Model file for the job. Use its own axes, mm. A direction names the side the tool comes from. Coordinates: 2 decimals unless noted, no trailing zeros. Loops run counter-clockwise (first coordinate to the right, second up) from the corner with the lowest first, then second, coordinate; pieces in that order, holes last. Notation, with made-up numbers: (2, 4.5) -> (6, 4.5) arc R33 ccw to (6, 42.5) -> close; hole circle Ø6 at (64.5, -21). An arc over 180 degrees is marked (long way). Use one line per item in the form item = value.
```python
from build123d import *

# Parameters (mm, degrees)
SKETCH1_W           = 100
SKETCH1_H           = 20
BOSS_EXTRUDE1_DEPTH = 3
SKETCH2_W           = 4.785100676
SKETCH2_H           = 2.523053084
CUT_EXTRUDE1_DEPTH  = 3


with BuildPart() as part:
    # Sketch1 → Boss-Extrude1 (new body)
    with BuildSketch(Plane(origin=(0, 0, 0), x_dir=(1, 0, 0), z_dir=(0, 1, 0))):
        with Locations((50, -10)):
            Rectangle(SKETCH1_W, SKETCH1_H)
    extrude(amount=BOSS_EXTRUDE1_DEPTH)

    # Sketch2 → Cut-Extrude1 (cut)
    with BuildSketch(Plane(origin=(0, 3, 0), x_dir=(1, 0, 0), z_dir=(0, 1, 0))):
        with BuildLine():
            ThreePointArc((41.05, -10), (40, -8.95), (38.95, -10))
            Line((38.95, -10), (41.05, -10))
        make_face()
        with BuildLine():
            Line((41.05, -10), (38.95, -10))
            ThreePointArc((38.95, -10), (40, -11.05), (41.05, -10))
        make_face()
        with BuildLine():
            ThreePointArc((31, -10), (30, -9), (29, -10))
            Line((29, -10), (31, -10))
        make_face()
        with BuildLine():
            Line((31, -10), (29, -10))
            ThreePointArc((29, -10), (30, -11), (31, -10))
        make_face()
        with Locations((30.05546257, -3.512455318)):
            Rectangle(SKETCH2_W, SKETCH2_H)
        with BuildLine():
            ThreePointArc((20.95, -10), (20, -9.05), (19.05, -10))
            Line((19.05, -10), (20.95, -10))
        make_face()
        with BuildLine():
            Line((20.95, -10), (19.05, -10))
            ThreePointArc((19.05, -10), (20, -10.95), (20.95, -10))
        make_face()
        with BuildLine():
            ThreePointArc((71.2, -10), (70, -8.8), (68.8, -10))
            Line((68.8, -10), (71.2, -10))
        make_face()
        with BuildLine():
            Line((71.2, -10), (68.8, -10))
            ThreePointArc((68.8, -10), (70, -11.2), (71.2, -10))
        make_face()
        with BuildLine():
            ThreePointArc((81.25, -10), (80, -8.75), (78.75, -10))
            Line((78.75, -10), (81.25, -10))
        make_face()
        with BuildLine():
            Line((81.25, -10), (78.75, -10))
            ThreePointArc((78.75, -10), (80, -11.25), (81.25, -10))
        make_face()
        with BuildLine():
            ThreePointArc((51.1, -10), (50, -8.9), (48.9, -10))
            Line((48.9, -10), (51.1, -10))
        make_face()
        with BuildLine():
            Line((51.1, -10), (48.9, -10))
            ThreePointArc((48.9, -10), (50, -11.1), (51.1, -10))
        make_face()
        with BuildLine():
            ThreePointArc((10.9, -10), (10, -9.1), (9.1, -10))
            Line((9.1, -10), (10.9, -10))
        make_face()
        with BuildLine():
            Line((10.9, -10), (9.1, -10))
            ThreePointArc((9.1, -10), (10, -10.9), (10.9, -10))
        make_face()
        with BuildLine():
            ThreePointArc((61.15, -10), (60, -8.85), (58.85, -10))
            Line((58.85, -10), (61.15, -10))
        make_face()
        with BuildLine():
            Line((61.15, -10), (58.85, -10))
            ThreePointArc((58.85, -10), (60, -11.15), (61.15, -10))
        make_face()
    extrude(amount=-CUT_EXTRUDE1_DEPTH, mode=Mode.SUBTRACT)


solid = part.part
```
Q1. Band-saw the part on A-A, the plane x = 40. Write the cut outline in (y, z).
Result:
outline = (0, 0) -> (3, 0) -> (3, 8.95) -> (0, 8.95) -> close; (0, 11.05) -> (3, 11.05) -> (3, 20) -> (0, 20) -> close
Q2. Band-saw the part on B-B, the plane y = 0.45. State how many separate pieces and enclosed holes the cut face has, and give its area (3 significant figures).
Result:
separate_pieces = 1
enclosed_holes = 9
area = 1,960 mm2
Q3. Which spindle directions (+Z, -Z, +X, -X, +Y, -Y) get a long thin tool onto all of the face, cutting with end or side? Do faces 1 (the face through (27.663, 2, 4)), 2 (the face through (100, 1, 10)). Say none if no direction does.
Result:
face_1 = +Y, -Y
face_2 = +Z, -Z, +X, +Y, -Y
Q4. Band-saw the part on D-D, the plane x = 70. Write the cut outline in (y, z).
Result:
outline = (0, 0) -> (3, 0) -> (3, 8.8) -> (0, 8.8) -> close; (0, 11.2) -> (3, 11.2) -> (3, 20) -> (0, 20) -> close
Q5. Wall check: line 1 along Z through (x, y) = (40, 1.55); line 2 along Z through (x, y) = (60, 1.35). Give the ranges that are in metal, low to high.
Result:
line_1 = 0 to 8.95, 11.05 to 20
line_2 = 0 to 8.85, 11.15 to 20
Q6. Mould opens along Z. For faces 3 (the face through (49, 1, 20)), 4 (the face through (0, 1, 10)), 5 (the face through (58.938, 1.521, 9.56)) say: released by +Z, released by -Z, zero draft, split by the parting line, or undercut.
Result:
face_3 = released by +Z
face_4 = zero draft
face_5 = undercut
